Work out the finished part from the listing and answer in its coordinate system (mm). Give positions to 0.01 mm unless a question says otherwise; leave off trailing zeros. Loops run counter-clockwise (first coordinate to the right, second up) from the corner with the lowest first, then second, coordinate; pieces in that order, holes last. Notation, with made-up numbers: (52, 64) - (78, 64) arc R15 cw to (78, 91) - close; hole circle Ø5 at (25, 20). An arc over 180 degrees is marked (long way). One line per question, with ' | ' between items.
from build123d import *

# Parameters (mm, degrees)
SKETCH1_W                      = 144
SKETCH1_H                      = 16
BOSS_EXTRUDE1_DEPTH            = 16
SKETCH2_W                      = 12.8
SKETCH2_H                      = 12.8
CUT_EXTRUDE1_DEPTH             = 145
F_3_7_3_7_DIAMETER_HOLE1_D     = 3.7
F_3_7_3_7_DIAMETER_HOLE1_DEPTH = 16
F_3_7_3_7_DIAMETER_HOLE2_D     = 3.7
F_3_7_3_7_DIAMETER_HOLE2_DEPTH = 16
FILLET1_R                      = 2


with BuildPart() as part:
    # Sketch1 → Boss-Extrude1 (new body)
    with BuildSketch(Plane(origin=(16, 0, 0), x_dir=(0, 0, -1), z_dir=(1, 0, 0))):
        with Locations((72, 8)):
            Rectangle(SKETCH1_W, SKETCH1_H)
    extrude(amount=-BOSS_EXTRUDE1_DEPTH)

    # Sketch2 → Cut-Extrude1 (cut, through all)
    with BuildSketch(Plane.XY):
        with Locations((9.6, 9.6)):
            Rectangle(SKETCH2_W, SKETCH2_H)
    extrude(amount=-CUT_EXTRUDE1_DEPTH, mode=Mode.SUBTRACT)

    # Ø3.7 (3.7) Diameter Hole1
    with Locations(Plane.ZY):
        with Locations((-24, 9.6), (-40, 9.6), (-56, 9.6), (-72, 9.6), (-88, 9.6), (-104, 9.6), (-120, 9.6), (-136, 9.6), (-8, 9.6)):
            Hole(F_3_7_3_7_DIAMETER_HOLE1_D / 2, depth=F_3_7_3_7_DIAMETER_HOLE1_DEPTH)

    # Ø3.7 (3.7) Diameter Hole2
    with Locations(Plane(origin=(0, 0, 0), x_dir=(-1, 0, 0), z_dir=(0, -1, 0))):
        with Locations((-9.6, 24), (-9.6, 40), (-9.6, 56), (-9.6, 72), (-9.6, 88), (-9.6, 104), (-9.6, 120), (-9.6, 136), (-9.6, 8)):
            Hole(F_3_7_3_7_DIAMETER_HOLE2_D / 2, depth=F_3_7_3_7_DIAMETER_HOLE2_DEPTH)

    # Fillet1
    fillet1_edges = [part.edges().sort_by_distance(p)[0] for p in [
        (16, 1.6, 0),
        (16, 1.6, -144),
        (1.6, 16, 0),
        (1.6, 16, -144),
    ]]
    fillet(fillet1_edges, radius=FILLET1_R)


solid = part.part
1. Find section A-A on z = -24. Write down the section's boundary in (x, y).
Evaluation:
outline: (0, 0) - (7.75, 0) - (7.75, 3.2) - (3.2, 3.2) - (3.2, 7.75) - (0, 7.75) - close; (0, 11.45) - (3.2, 11.45) - (3.2, 16) - (0, 16) - close; (11.45, 0) - (16, 0) - (16, 3.2) - (11.45, 3.2) - close
2. Determine the mould class of faces 1 (the flat face through (4, 2, 0)), 2 (the cylindrical face through (9.199, 1.622, -70.194)), 3 (the flat face through (16, 2, -71)) for opening direction Z: +Z half, -Z half, draft (parallel to the pull), parting line (faces both ways), or undercut.
Evaluation:
face 1: +Z half | face 2: undercut | face 3: draft
3. Find section B-B on x = 1.5. State how many separate pieces and enclosed holes the cut face has, then the cut area to 3 significant figures.
Evaluation:
separate pieces: 1 | enclosed holes: 9 | area: 2,210 mm2
4. Flat-ended cylindrical pins translate along their axes: pin 1 (2 mm diameter, centred on y = 9.6, z = -72, fed in from -X); pin 2 (3 mm diameter, centred on x = 2, z = -25.5, fed in from -Y); pin 3 (5 mm diameter, centred on y = 9.6, z = -8, fed in from +X); pin 4 (4.5 mm diameter, centred on x = 9.6, z = -40, fed in from +Y). Find the tip coordinate at first contact, or state that the pin passes through.
Evaluation:
pin 1: through | pin 2: y = 0 | pin 3: x = 3.2 | pin 4: y = 3.2
5. Consider L1, parallel to Y at x = 0.85, z = -40; L2, parallel to Z at x = 1.5, y = 14.25. Determine where each line is inside the solid, lowest interval first.
Evaluation:
L1: 0 to 7.75, 11.45 to 16 | L2: -143.98 to -0.02
